Autodesk Inventor part; units mm, degrees
ref_plane "YZ Plane" through (0, 0, 0) normal (1, 0, 0) x (0, 1, 0)
ref_plane "XZ Plane" through (0, 0, 0) normal (0, 1, 0) x (-1, 0, 0)
ref_plane "XY Plane" through (0, 0, 0) normal (0, 0, 1) x (1, 0, 0)
sketch "Sketch1" plane through (0, 0, 0) normal (0, 1, 0) x (-1, 0, 0)
  line L0 (-36.5, -40) -> (-36.5, 40)
  line L1 (36.5, 40) -> (36.5, -40)
  line L2 (-36.5, 40) -> (36.5, -40) construction
  line L3 (36.5, 40) -> (-36.5, -40) construction
  line L4 (36.5, 40) -> (36.5, 13)
  line L5 (-36.5, 40) -> (36.5, 40)
  line L6 (-36.5, -40) -> (-9.5, -40)
  line L7 (-36.5, -40) -> (18.5, -40)
  line L8 (36.5, -40) -> (-36.5, -40)
  line L9 (36.5, -40) -> (28.5, -40)
  line L10 (28.5, -40) -> (28.5, -32)
  line L11 (28.5, -32) -> (36.5, -32)
  line L12 (36.5, -32) -> (36.5, -40)
  line L13 (36.5, 40) -> (28.5, 40)
  line L14 (28.5, 40) -> (28.5, 32)
  line L15 (28.5, 32) -> (36.5, 32)
  line L16 (36.5, 32) -> (36.5, 40)
  line L17 (-36.5, 40) -> (-28.5, 40)
  line L18 (-28.5, 40) -> (-28.5, 32)
  line L19 (-28.5, 32) -> (-36.5, 32)
  line L20 (-36.5, 32) -> (-36.5, 40)
  line L21 (-36.5, -40) -> (-28.5, -40)
  line L22 (-28.5, -40) -> (-28.5, -32)
  line L23 (-28.5, -32) -> (-36.5, -32)
  line L24 (-36.5, -32) -> (-36.5, -40)
  dimension "d0" = 73
  dimension "d1" = 80
  dimension "d10" = 8
  dimension "d11" = 8
  dimension "d12" = 8
  dimension "d13" = 8
  dimension "d14" = 8
  dimension "d15" = 8
  dimension "d16" = 8
  dimension "d17" = 8
extrude "Extrusion1" add sketch "Sketch1" along normal blind 100 contours L0 L23 L22 L6 | L0 L5 L18 L19 | L10 L11 L1 L8 | L5 L1 L15 L14
sketch "Sketch2" plane through (0, 100, 0) normal (0, 1, 0) x (1, 0, 0)
  line L0 (-36.5, -40) -> (-28.5, -40)
  line L1 (-28.5, 32) -> (-28.5, 40)
  line L2 (-36.5, -40) -> (-28.5, -40)
  line L3 (-28.5, -40) -> (-28.5, 40)
  line L4 (-28.5, 40) -> (-36.5, 40)
  line L5 (-36.5, 40) -> (-36.5, -40)
  line L6 (-36.5, -32) -> (-36.5, -40)
  line L7 (36.5, -40) -> (36.5, -32)
  line L8 (-36.5, -40) -> (36.5, -40)
  line L9 (36.5, -40) -> (36.5, -32)
  line L10 (36.5, -32) -> (-36.5, -32)
  line L11 (-36.5, -32) -> (-36.5, -40)
  line L12 (28.5, -32) -> (28.5, -40)
  line L13 (36.5, 40) -> (28.5, 40)
  line L14 (28.5, -32) -> (36.5, -32)
  line L15 (36.5, -32) -> (36.5, 40)
  line L16 (36.5, 40) -> (28.5, 40)
  line L17 (28.5, 40) -> (28.5, -32)
  line L18 (-28.5, 32) -> (-28.5, 40)
  line L19 (28.5, 40) -> (28.5, 32)
  line L20 (-28.5, 40) -> (28.5, 40)
  line L21 (28.5, 40) -> (28.5, 32)
  line L22 (28.5, 32) -> (-28.5, 32)
  line L23 (-28.5, 32) -> (-28.5, 40)
  point P0 (0, 0)
extrude "Extrusion2" add sketch "Sketch2" along normal blind 8 contours L5 L10 L3 L0 | L3 L10 L12 L8 | L5 L4 L1 L3 L10 | L12 L10 L7 L8 | L1 L20 L17 L22 | L17 L13 L15 L10
sketch "Sketch3" plane through (0, 108, 0) normal (0, 1, 0) x (1, 0, 0)
  line L0 (28.5, -32) -> (-28.5, -32)
  line L1 (28.5, 32) -> (36.5, 32)
  line L2 (-28.5, -32) -> (28.5, -32)
  line L3 (28.5, -32) -> (28.5, 32)
  line L4 (28.5, 32) -> (-28.5, 32)
  line L5 (-28.5, 32) -> (-28.5, -32)
  line L6 (32.5, 36) -> (32.5, -36)
  line L7 (32.5, -36) -> (-32.5, -36)
  line L8 (-32.5, -36) -> (-32.5, 36)
  line L9 (-32.5, 36) -> (32.5, 36)
  point P0 (0, 0)
  dimension "d22" = 4
extrude "Extrusion3" cut sketch "Sketch3" against normal blind 3
fillet "Fillet1" radius 2 8 edges at (32.5, 100, 32) (-28.5, 100, -36) (-28.5, 100, 36) (28.5, 100, -36) (-32.5, 100, 32) (-32.5, 100, -32) (28.5, 100, 36) (32.5, 100, -32)
fillet "Fillet2" radius 2 4 edges at (-36.5, 108, 0) (0, 108, 40) (36.5, 108, 0) (0, 108, -40)
properties part number "Hood_base"
Here's how the part is built. I have some questions about the finished solid (model axes, mm). A direction names the side the tool comes from. Coordinates: 2 decimals unless noted, no trailing zeros. Write each loop counter-clockwise with the first axis right and the second up, starting at its lowest first coordinate (ties: lowest second). Pieces come first, ordered by that corner, then holes. Notation, with made-up numbers: M 10,-31.75 L 47,-31.75 A23 ccw 47,-6.75 Z; hole C 88,53 d9. An arc over 180 degrees is marked long. Answer as CSV lines item,"result". Start each with the question number.
Q1. Will these pins go through, and if not, where does the flat tip stop? pin 1 Ø1.5 at (y, z) = (107, 6) entering from +X; pin 2 Ø9 at (x, z) = (-33.5, -13.5) entering from -Y.
Q2. For faces 4 (the flat face through (28.5, 103, 0)), 5 (the flat face through (-0.2, 105, -32.2)), 6 (the flat face through (-33, 108, 0)), 7 (the flat face through (28.5, 48, 36)), 8 (the flat face through (-33, 100, 0)), which set-ups out of +Z, -Z, +X, -X, +Y, -Y let a thin tool reach every point of the face, with its end or its side?
Q3. Suppose I cut it at C-C, the plane x = -14.5. List the corners of the cut face in (y, z) for me.
Q4. Suppose I cut it at B-B, the plane z = -14.5. List the corners of the cut face in (x, y) for me, then the cut area to 3 significant figures.
Q5. Suppose I cut it at A-A, the plane y = 47. List the corners of the cut face in (x, z) for me, then the cut area to 3 significant figures.
Q6. If we mould it in two halves opening along X, with no side actions, what happens to faces 1 (the flat face through (0, 107, -36)), 2 (the flat face through (-32, 48, -32)), 3 (the flat face through (-36.5, 61, -33))? For each: pulls with the +X half, pulls with the -X half, needs draft (parallel to the pull), parting line crosses it, or undercut.
Q7. I need wall thicknesses on probe 1 along X at (y, z) = (37, -32.5); probe 2 along Z at (x, y) = (31.5, 32.5); probe 3 along Y at (x, z) = (-30.5, -15). Which ranges of each line are inside material? Lowest first, please. Write a range as [from, to].
Entries:
1,pin 1,"stops at x = 36.48"
1,pin 2,"stops at y = 100"
2,face 4,"+Y, -Y"
2,face 5,"+Y"
2,face 6,"+Z, -Z, +X, -X, +Y"
2,face 7,"+Z, -Z, -Y"
2,face 8,"+X, -X, -Y"
3,outline,"M 100,-40 L 106,-40 A2 ccw 108,-38 L 108,-36 L 105,-36 L 105,-32 L 100,-32 Z; M 100,32 L 105,32 L 105,36 L 108,36 L 108,38 A2 ccw 106,40 L 100,40 Z"
4,outline,"M -36.5,100 L -28.5,100 L -28.5,105 L -32.5,105 L -32.5,108 L -34.5,108 A2 ccw -36.5,106 Z; M 28.5,100 L 36.5,100 L 36.5,106 A2 ccw 34.5,108 L 32.5,108 L 32.5,105 L 28.5,105 Z"
4,area,"102 mm²"
5,outline,"M -36.5,-40 L -28.5,-40 L -28.5,-32 L -36.5,-32 Z; M -36.5,32 L -28.5,32 L -28.5,40 L -36.5,40 Z; M 28.5,-40 L 36.5,-40 L 36.5,-32 L 28.5,-32 Z; M 28.5,32 L 36.5,32 L 36.5,40 L 28.5,40 Z"
5,area,"256 mm²"
6,face 1,"undercut"
6,face 2,"needs draft"
6,face 3,"pulls with the -X half"
7,probe 1,"x = [-36.5, -28.5], [28.5, 36.5]"
7,probe 2,"z = [-40, -32], [32, 40]"
7,probe 3,"y = [100, 105]"
